Geometry check sheet. Reference: the model listing, model coordinates, mm. Face numbers are marked on the shaded views. A direction names the side the tool comes from. Round coordinates to 2 decimals unless told otherwise and drop trailing zeros. Order: outer loops, then holes, each group sorted by start corner. A loop starts at its lowest first (then second) coordinate and runs counter-clockwise, first axis right, second up. Notation, with made-up numbers: (-4.5, 75.5) -> (29.5, 75.5) arc R26 cw to (29.5, 93.5) -> close; hole circle Ø4 at (-25.75, 20.5). An arc over 180 degrees is marked (long way). Use a Markdown table: item, result. Add a question column.
Item 1: Mould release check, pull along X, two halves, no side actions. Record for the marked faces 4, 5 and 6: pulls with the +X half, pulls with the -X half, needs draft (parallel to the pull), parting line crosses it, or undercut.
Item 2: Set-up check for the marked faces 1, 2 and 3: record each of +Z, -Z, +X, -X, +Y, -Y from which the full face is reachable in a straight line by a thin tool's end or side.
Item 3: Sectioned sample at C-C, the plane x = -14. Record the cut outline in (y, z), and give its area (3 significant figures).
Item 4: Sectioned sample at A-A, the plane y = -13.5. Record the cut outline in (x, z), and give its area (3 significant figures).
Item 5: Material ranges on probe 1 along X at (y, z) = (-21, 5); probe 2 along X at (y, z) = (-8, 63); probe 3 along Y at (x, z) = (-5.5, 58.5), recorded low to high. Write a range as [from, to].
Item 6: Sectioned sample at B-B, the plane z = 62. Record the cut outline in (x, y), and give its area (3 significant figures).
Item 7: Gauge pin test, flat ends, axial feed: pin 1 Ø12 at (x, y) = (-17, -6.5) entering from -Z; pin 2 Ø3 at (x, y) = (-14.5, -23.5) entering from +Z; pin 3 Ø10 at (x, y) = (-11.33, -23.28) entering from +Z; pin 4 Ø10 at (y, z) = (-24, 47) entering from +X. Record the tip position at first contact, or that the pin passes through.
Item 8: Sectioned sample at D-D, the plane y = -2.5. Record the cut outline in (x, z).
from build123d import *

# Parameters (mm, degrees)
F0_W      = 50.8
F0_H      = 6.35
F1_DEPTH  = 31.75
F2_W      = 50.8
F2_H      = 12.7
F3_DEPTH  = 69.85
F4_R      = 4.1454227759
F4_R_2    = 3.8275327049
F5_DEPTH  = 12.7
F7_DEPTH  = 12.7
F8_R      = 5.3504269389
F9_DEPTH  = 12.7
F10_DEPTH = 12.7


with BuildPart() as f1:
    # F0 (on Front) → F1 (new body)
    with BuildSketch(Plane.XZ):
        with Locations((2.6147060619, 3.175)):
            Rectangle(F0_W, F0_H)
    extrude(amount=F1_DEPTH)

    # F2 (on face) → F3 (join)
    with BuildSketch(Plane.XY.offset(6.35)):
        with Locations((2.6147060619, -6.35)):
            Rectangle(F2_W, F2_H)
    extrude(amount=F3_DEPTH)

    # F4 (on face) → F5 (cut)
    with BuildSketch(Plane.XY.offset(6.35)):
        with Locations((15.8469081592, -23.275712505)):
            Circle(F4_R)
        with Locations((-11.3311024653, -23.275712505)):
            Circle(F4_R_2)
        with BuildLine():
            ThreePointArc((-12.9734249786, -31.75), (-18.8152455834, -29.3930620602), (-22.7852939381, -24.5021786541))
            Line((-22.7852939381, -24.5021786541), (-22.7852939381, -31.75))
            Line((-22.7852939381, -31.75), (-12.9734249786, -31.75))
        make_face()
        with BuildLine():
            ThreePointArc((28.0147060619, -24.5021786541), (24.4846674342, -29.0776682905), (19.3607117981, -31.75))
            Line((19.3607117981, -31.75), (28.0147060619, -31.75))
            Line((28.0147060619, -31.75), (28.0147060619, -24.5021786541))
        make_face()
    extrude(amount=-F5_DEPTH, mode=Mode.SUBTRACT)

    # F6 (on face) → F7 (cut)
    with BuildSketch(Plane.XZ.offset(12.7)):
        with BuildLine():
            Line((-22.7852939381, 76.2), (-22.7852939381, 6.35))
            ThreePointArc((-22.7852939381, 6.35), (-13.8298680574, 12.9622223367), (-10.3186676279, 23.5259626061))
            Line((-10.3186676279, 23.5259626061), (-10.3186676279, 76.2))
            Line((-10.3186676279, 76.2), (-22.7852939381, 76.2))
        make_face()
        with BuildLine():
            ThreePointArc((15.0813323721, 23.5259626061), (19.1005030761, 13.0950196253), (28.0147060619, 6.35))
            Line((28.0147060619, 6.35), (28.0147060619, 76.2))
            Line((28.0147060619, 76.2), (15.0813323721, 76.2))
            Line((15.0813323721, 76.2), (15.0813323721, 23.5259626061))
        make_face()
    extrude(amount=-F7_DEPTH, mode=Mode.SUBTRACT)

    # F8 (on face) → F9 (join)
    with BuildSketch(Plane.XZ.offset(12.7)):
        with BuildLine():
            Line((15.0813323721, 62.8083311773), (15.0813323721, 64.1052759432))
            ThreePointArc((15.0813323721, 64.1052759432), (2.3813323721, 76.1733485482), (-10.3186676279, 64.1052759432))
            Line((-10.3186676279, 64.1052759432), (-10.3186676279, 62.8083311773))
            ThreePointArc((-10.3186676279, 62.8083311773), (2.3813323721, 50.7402585723), (15.0813323721, 62.8083311773))
        make_face()
        with Locations((2.3813323721, 63.4568035603)):
            Circle(F8_R, mode=Mode.SUBTRACT)
    extrude(amount=F9_DEPTH)

    # F10 (cut): faces of the model
    f10_faces = [f1.faces().sort_by_distance(p)[0] for p in [
        (14.8000065201, -12.7, 70.1526379716),
        (2.3813323721, -12.7, 63.4568035603),
    ]]
    extrude(f10_faces, amount=-F10_DEPTH, mode=Mode.SUBTRACT)


solid = f1.part
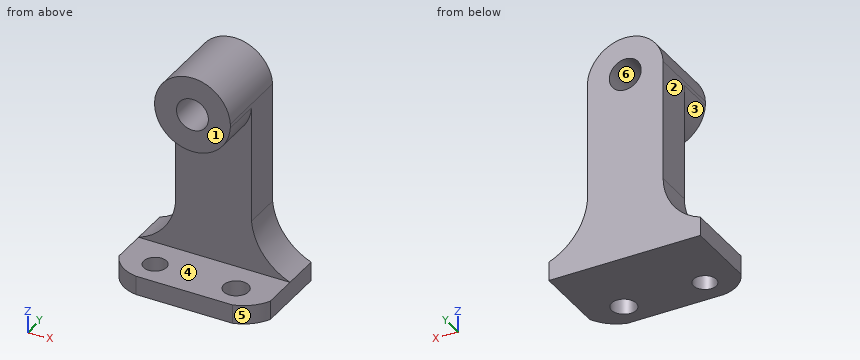
Found:
| question | item | result |
|---|---|---|
| 1 | face 4 | needs draft |
| 1 | face 5 | pulls with the +X half |
| 1 | face 6 | undercut |
| 2 | face 1 | +Z, +X, -X, -Y |
| 2 | face 2 | +Z, -X, +Y, -Y |
| 2 | face 3 | -Y |
| 3 | outline | (-31.57, 0) -> (-26.02, 0) -> (-26.02, 6.35) -> (-31.57, 6.35) -> close; (-20.53, 0) -> (0, 0) -> (0, 12.73) -> (-12.7, 12.73) -> (-12.7, 6.35) -> (-20.53, 6.35) -> close |
| 3 | area | 247 mm2 |
| 4 | outline | (-22.79, 0) -> (28.01, 0) -> (28.01, 6.35) -> (-22.79, 6.35) -> close; (-10.32, 62.81) arc R12.72 ccw to (15.08, 62.81) -> (15.08, 64.11) arc R12.72 ccw to (-10.32, 64.11) -> close; hole circle Ø10.7 at (2.38, 63.46) |
| 4 | area | 741 mm2 |
| 5 | probe 1 | x = [-22.79, -14.41], [-8.25, 12.38], [19.31, 28.01] |
| 5 | probe 2 | x = [-10.32, -2.95], [7.71, 15.08] |
| 5 | probe 3 | y = [-25.4, 0] |
| 6 | outline | (-10.32, -12.7) -> (-10.25, -12.7) -> (-10.25, -25.4) -> (-2.77, -25.4) -> (-2.77, 0) -> (-10.32, 0) -> close; (7.53, -25.4) -> (15.01, -25.4) -> (15.01, -12.7) -> (15.08, -12.7) -> (15.08, 0) -> (7.53, 0) -> close |
| 6 | area | 382 mm2 |
| 7 | pin 1 | stops at z = 0 |
| 7 | pin 2 | stops at z = 6.35 |
| 7 | pin 3 | stops at z = 72.72 |
| 7 | pin 4 | stops at x = 7.9 |
| 8 | outline | (-22.79, 0) -> (28.01, 0) -> (28.01, 6.35) arc R20.39 cw to (15.08, 23.53) -> (15.08, 64.11) arc R12.72 ccw to (-10.32, 64.11) -> (-10.32, 23.53) arc R18.42 cw to (-22.79, 6.35) -> close; hole circle Ø10.7 at (2.38, 63.46) |
